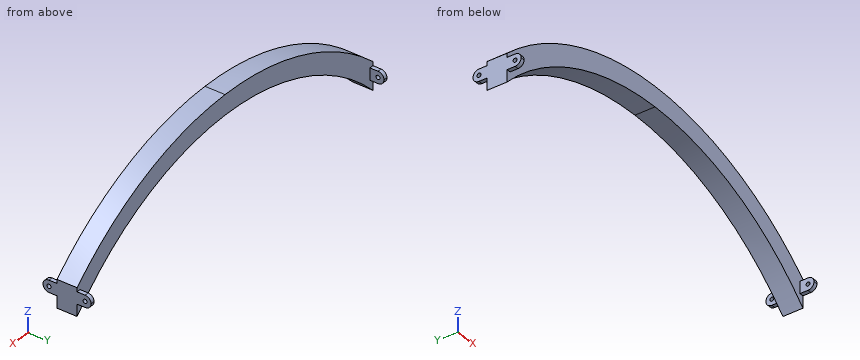
```python
from build123d import *

# Parameters (mm, degrees)
F1_W     = 50
F1_H     = 50
F3_W     = 64.371526
F3_H     = 133.521259
F4_DEPTH = 91
F5_R     = 5
F6_DEPTH = 10


with BuildPart() as f2:
    # F2: sweep along a path in F0
    with BuildLine(Plane.XZ) as f2_path:
        ThreePointArc((0, 690), (272.034172, 634.111512), (500, 475.499737))
    # F1 (on Right) → F2 (sweep)
    with BuildSketch(Plane.YZ):
        with Locations((-25, 715)):
            Rectangle(F1_W, F1_H)
    sweep(path=f2_path.line)

    # F3 (on Front) → F4 (cut)
    with BuildSketch(Plane.XZ):
        with Locations((532.185763, 516.52947)):
            Rectangle(F3_W, F3_H)
    extrude(amount=F4_DEPTH, mode=Mode.SUBTRACT)

    # F5 (on face) → F6 (join)
    with BuildSketch(Plane.YZ.offset(500)):
        with BuildLine():
            Line((-50, 505.527268), (-50, 535.527268))
            Line((-50, 535.527268), (-70, 535.527268))
            ThreePointArc((-70, 535.527268), (-80.606602, 531.13387), (-85, 520.527268))
            ThreePointArc((-85, 520.527268), (-80.606602, 509.920666), (-70, 505.527268))
            Line((-70, 505.527268), (-50, 505.527268))
        make_face()
        with Locations((-70, 520.527268)):
            Circle(F5_R, mode=Mode.SUBTRACT)
        with BuildLine():
            Line((20, 535.527268), (0, 535.527268))
            Line((0, 535.527268), (0, 505.527268))
            Line((0, 505.527268), (20, 505.527268))
            ThreePointArc((20, 505.527268), (30.606602, 509.920666), (35, 520.527268))
            ThreePointArc((35, 520.527268), (30.606602, 531.13387), (20, 535.527268))
        make_face()
        with Locations((20, 520.527268)):
            Circle(F5_R, mode=Mode.SUBTRACT)
    extrude(amount=-F6_DEPTH)

    # F7: F2 across face


with BuildPart() as f2_1:
    add(f2.part)
    add(f2.part.mirror(Plane(origin=(0, -25, 715), x_dir=(0, -1, 0), z_dir=(-1, 0, 0))))


solid = f2_1.part
```
Source: CAD feature listing. Evaluate the final solid. Frame: model axes, mm. Give positions to 0.01 mm unless a question says otherwise; leave off trailing zeros. Order: outer loops, then holes, each group sorted by start corner. A loop starts at its lowest first (then second) coordinate and runs counter-clockwise, first axis right, second up. Notation, with made-up numbers: (-15, 40.5) -> (22, 40.5) arc R17 cw to (22, 56.5) -> close; hole circle Ø8 at (-1, -34.75). An arc over 180 degrees is marked (long way). Use a Markdown table: item, result.
Q1. Material intervals for line 1 (Z direction, x = -493, y = -70); line 2 (Y direction, x = 21.5, z = 716); line 3 (X direction, y = -26, z = 630), sorted ascending. Write a range as [from, to].
A:
| item | result |
|---|---|
| line 1 | [505.53, 515.53], [525.53, 535.53] |
| line 2 | [-50, 0] |
| line 3 | [-388.2, -281.42], [281.42, 388.2] |
Q2. First-contact query: P1, Ø5, axis at x = 494.5, y = -65, coming from the -Z side; P2, Ø11, axis at x = 496.5, y = 13, coming from the +Z side; P3, Ø3, axis at y = -14, z = 667.5, coming from the +X side; P4, Ø11.5, axis at y = -70, z = 520.53, coming from the -X side. Flat tips, straight axial feed; report the tip coordinate or a pass-through.
A:
| item | result |
|---|---|
| P1 | z = 505.53 |
| P2 | z = 535.53 |
| P3 | x = 322.56 |
| P4 | x = -500 |
Q3. Section A-A (z = 650). Return the cut outline in (x, y), and give its area (3 significant figures).
A:
| item | result |
|---|---|
| outline | (-353.69, -50) -> (-231.52, -50) -> (-231.52, 0) -> (-353.69, 0) -> close; (231.52, -50) -> (353.69, -50) -> (353.69, 0) -> (231.52, 0) -> close |
| area | 12,200 mm^2 |
Q4. Section C-C (x = 76). Return the cut outline in (y, z).
A:
| item | result |
|---|---|
| outline | (-50, 685.8) -> (0, 685.8) -> (0, 736.09) -> (-50, 736.09) -> close |
Q5. Section B-B (x = 401). Return the cut outline in (y, z).
A:
| item | result |
|---|---|
| outline | (-50, 561.51) -> (0, 561.51) -> (0, 621.93) -> (-50, 621.93) -> close |
